from build123d import *

# Parameters (mm, degrees)
SKETCH_1_W          = 14.4
SKETCH_1_H          = 12.4
SKETCH_1_R          = 3.5
SKETCH_1_R_2        = 0.4
EXTRUDE_1_DEPTH     = 1.7
SKETCH_2_W          = 10.8
SKETCH_2_H          = 11.5
SKETCH_2_W_2        = 6.8
SKETCH_2_H_2        = 7.5
EXTRUDE_1_2_DEPTH   = 4
FILLET_1_R          = 1.5
SKETCH_3_W          = 2.2
SKETCH_3_H          = 2
SKETCH_3_W_2        = 2.6
CUT_EXTRUDE_1_DEPTH = 1.5
SKETCH_4_R          = 0.4
CUT_EXTRUDE_2_DEPTH = 3


with BuildPart() as part:
    # 草图1 → Extrude 1 (new body)
    with BuildSketch(Plane(origin=(0, 0, 0), x_dir=(1, 0, 0), z_dir=(0, 1, 0))):
        Rectangle(SKETCH_1_W, SKETCH_1_H)
        with Locations(Location((0, 0, 0), (0, 0, 270))):
            Circle(SKETCH_1_R, mode=Mode.SUBTRACT)
        with Locations(Location((5.45, -4.95, 0), (0, 0, 270))):
            Circle(SKETCH_1_R_2, mode=Mode.SUBTRACT)
        with Locations(Location((-5.45, -4.95, 0), (0, 0, 270))):
            Circle(SKETCH_1_R_2, mode=Mode.SUBTRACT)
        with Locations(Location((5.45, 4.95, 0), (0, 0, 270))):
            Circle(SKETCH_1_R_2, mode=Mode.SUBTRACT)
        with Locations(Location((-5.45, 4.95, 0), (0, 0, 270))):
            Circle(SKETCH_1_R_2, mode=Mode.SUBTRACT)
    extrude(amount=EXTRUDE_1_DEPTH)

    # 草图2 → Extrude 1 2 (add)
    with BuildSketch(Plane.XZ):
        with Locations((0, 0.35)):
            Rectangle(SKETCH_2_W, SKETCH_2_H)
        with Locations((0, 0.35)):
            Rectangle(SKETCH_2_W_2, SKETCH_2_H_2, mode=Mode.SUBTRACT)
    extrude(amount=EXTRUDE_1_2_DEPTH)

    # 圆角1
    fillet_1_edges = [part.edges().sort_by_distance(p)[0] for p in [
        (3.4, -2, -3.4),
        (-3.4, -2, -3.4),
    ]]
    fillet(fillet_1_edges, radius=FILLET_1_R)

    # 草图3 → 切除-拉伸1 (cut)
    with BuildSketch(Plane.XZ.offset(4)):
        with Locations((-2.3, 5.1)):
            Rectangle(SKETCH_3_W, SKETCH_3_H)
        with Locations((2.3, 5.1)):
            Rectangle(SKETCH_3_W, SKETCH_3_H)
        with Locations((0, -4.4)):
            Rectangle(SKETCH_3_W_2, SKETCH_3_H)
    extrude(amount=-CUT_EXTRUDE_1_DEPTH, mode=Mode.SUBTRACT)

    # 草图4 → 切除-拉伸2 (cut)
    with BuildSketch(Plane.XZ.offset(4)):
        with Locations(Location((-3.9, -4.15, 0), (0, 0, 270))):
            Circle(SKETCH_4_R)
        with Locations(Location((3.9, -4.15, 0), (0, 0, 270))):
            Circle(SKETCH_4_R)
        with Locations(Location((0, 5.1, 0), (0, 0, 270))):
            Circle(SKETCH_4_R)
    extrude(amount=-CUT_EXTRUDE_2_DEPTH, mode=Mode.SUBTRACT)


solid = part.part
Geometry check sheet. Reference: the model listing, model coordinates, mm. A direction names the side the tool comes from. Round coordinates to 2 decimals unless told otherwise and drop trailing zeros. Loops run counter-clockwise (first coordinate to the right, second up) from the corner with the lowest first, then second, coordinate; pieces in that order, holes last.
Item 1: Gauge pin test, flat ends, axial feed: pin 1 (1 mm diameter, centred on x = -2.5, y = -3.5, fed in from -Z); pin 2 (1.6 mm diameter, centred on x = -2.5, z = 5.5, fed in from -Y); pin 3 (1.2 mm diameter, centred on y = -3.5, z = 5, fed in from +X). Record the tip position at first contact, or that the pin passes through.
Item 2: Thickness scan on line 1 (Z direction, x = -5.45, y = 1.25); line 2 (X direction, y = -3.3, z = 5.1); line 3 (X direction, y = -2.3, z = -4.15). Record the ranges inside material, lowest first.
Item 3: Cross-section at D-D on z = -4.95. Record the boundary of the cut face in (x, y), then the cut area to 3 significant figures.
Item 4: Cross-section at A-A on y = -0.35. Record the boundary of the cut face in (x, z).
Item 5: Cross-section at C-C on x = 4.75. Record the boundary of the cut face in (y, z).
Item 6: Access from +Z, -Z, +X, -X, +Y, -Y to the whole of each face (thin tool, end or side, straight path). Record for faces 1 (the flat face through (2, -2.5, 5)), 2 (the flat face through (0, -2, 6.1)), 3 (the flat face through (0, -2, -5.4)).
Item 7: Cross-section at B-B on z = 0. Record the boundary of the cut face in (x, y).
Answer sheet:
1. pin 1: stops at z = -5.4
1. pin 2: stops at y = -2.5
1. pin 3: stops at x = 5.4
2. line 1: z = -6.2 to -5.35, -4.55 to 4.55, 5.35 to 6.2
2. line 2: x = -5.4 to -3.4, -1.2 to -0.4, 0.4 to 1.2, 3.4 to 5.4
2. line 3: x = -5.4 to -4.3, -3.5 to 3.5, 4.3 to 5.4
3. outline: (-7.2, 0) - (-5.85, 0) - (-5.85, 1.7) - (-7.2, 1.7) - close; (-5.4, -4) - (-1.3, -4) - (-1.3, -2.5) - (1.3, -2.5) - (1.3, -4) - (5.4, -4) - (5.4, 0) - (5.05, 0) - (5.05, 1.7) - (-5.05, 1.7) - (-5.05, 0) - (-5.4, 0) - close; (5.85, 0) - (7.2, 0) - (7.2, 1.7) - (5.85, 1.7) - close
3. area: 61.1 mm2
4. outline: (-5.4, -5.4) - (5.4, -5.4) - (5.4, 6.1) - (-5.4, 6.1) - close; hole (-3.4, -1.9) arc R1.5 ccw to (-1.9, -3.4) - (1.9, -3.4) arc R1.5 ccw to (3.4, -1.9) - (3.4, 4.1) - (-3.4, 4.1) - close
5. outline: (-4, -5.4) - (0, -5.4) - (0, -6.2) - (1.7, -6.2) - (1.7, 6.2) - (0, 6.2) - (0, 6.1) - (-4, 6.1) - close
6. face 1: +Z, -Y
6. face 2: +Z, +X, -X, -Y
6. face 3: -Z, +X, -X, -Y
7. outline: (-7.2, 0) - (-5.4, 0) - (-5.4, -4) - (-3.4, -4) - (-3.4, 0) - (-3.5, 0) - (-3.5, 1.7) - (-7.2, 1.7) - close; (3.4, -4) - (5.4, -4) - (5.4, 0) - (7.2, 0) - (7.2, 1.7) - (3.5, 1.7) - (3.5, 0) - (3.4, 0) - close
